from build123d import *

# Parameters (mm, degrees)
SKETCH1_W           = 28
SKETCH1_H           = 30
BOSS_EXTRUDE1_DEPTH = 12
SKETCH2_R           = 2.25
CUT_EXTRUDE1_DEPTH  = 36.213633723
SKETCH4_W           = 28
SKETCH4_H           = 15
CUT_EXTRUDE3_DEPTH  = 24.769728648
CUT_EXTRUDE4_DEPTH  = 5


with BuildPart() as part:
    # Sketch1 → Boss-Extrude1 (new body)
    with BuildSketch(Plane(origin=(0, 0, 0), x_dir=(1, 0, 0), z_dir=(0, 1, 0))):
        Rectangle(SKETCH1_W, SKETCH1_H)
        with BuildLine():
            Line((-1.590990258, -9.090990258), (0, -10.681980515))
            Line((0, -10.681980515), (1.590990258, -9.090990258))
            ThreePointArc((1.590990258, -9.090990258), (0, -5.25), (-1.590990258, -9.090990258))
        make_face(mode=Mode.SUBTRACT)
        with BuildLine():
            Line((-1.590990258, 5.909009742), (0, 4.318019485))
            Line((0, 4.318019485), (1.590990258, 5.909009742))
            ThreePointArc((1.590990258, 5.909009742), (0, 9.75), (-1.590990258, 5.909009742))
        make_face(mode=Mode.SUBTRACT)
    extrude(amount=BOSS_EXTRUDE1_DEPTH)

    # Sketch2 → Cut-Extrude1 (cut, through all)
    with BuildSketch(Plane.XY.offset(15)):
        with Locations((-9, 6)):
            Circle(SKETCH2_R)
        with Locations((9, 6)):
            Circle(SKETCH2_R)
    extrude(amount=-CUT_EXTRUDE1_DEPTH, mode=Mode.SUBTRACT)

    # Sketch4 → Cut-Extrude3 (cut, through all)
    with BuildSketch(Plane(origin=(0, 12, 0), x_dir=(1, 0, 0), z_dir=(0, 1, 0))):
        with Locations((0, -7.5)):
            Rectangle(SKETCH4_W, SKETCH4_H)
    extrude(amount=-CUT_EXTRUDE3_DEPTH, mode=Mode.SUBTRACT)

    # Sketch5 → Cut-Extrude4 (cut)
    with BuildSketch(Plane(origin=(0, 12, 0), x_dir=(1, 0, 0), z_dir=(0, 1, 0))):
        with BuildLine():
            Line((-2.828427125, 4.671572875), (0, 1.843145751))
            Line((0, 1.843145751), (2.828427125, 4.671572875))
            ThreePointArc((2.828427125, 4.671572875), (0, 11.5), (-2.828427125, 4.671572875))
        make_face()
    extrude(amount=-CUT_EXTRUDE4_DEPTH, mode=Mode.SUBTRACT)


solid = part.part
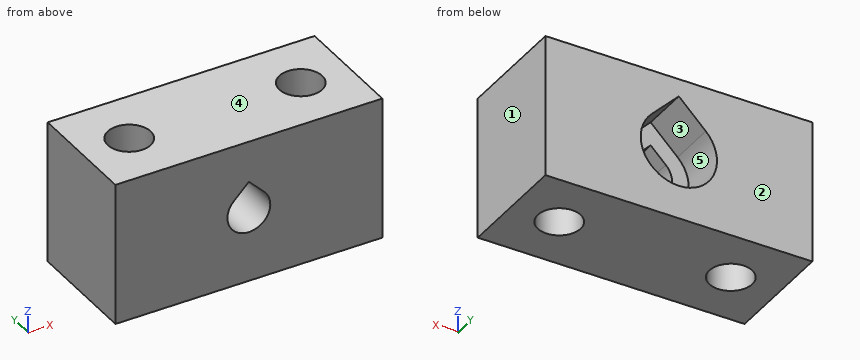
Here's how the part is built. I have some questions about the finished solid (model axes, mm). Face numbers are marked on the shaded views. A direction names the side the tool comes from. Give positions to 0.01 mm unless a question says otherwise; leave off trailing zeros. Order: outer loops, then holes, each group sorted by start corner. A loop starts at its lowest first (then second) coordinate and runs counter-clockwise, first axis right, second up. Notation, with made-up numbers: (-10, -27) -> (15, -27) arc R32 ccw to (15, 5) -> close; hole circle Ø9 at (23.25, 69.5). An arc over 180 degrees is marked (long way). Use a Markdown table: item, result. Add a question column.
Item 1: If we mould it in two halves opening along X, with no side actions, what happens to the marked faces 1, 2 and 3? For each: pulls with the +X half, pulls with the -X half, needs draft (parallel to the pull), parting line crosses it, or undercut.
Item 2: Imagine slicing it at D-D on z = -12.25. Please give me the cut outline in (x, y).
Item 3: Imagine slicing it at C-C on z = -7.5. Please give me the cut outline in (x, y).
Item 4: Will this pin go through, and if not, where does the flat tip stop? pin 1 (4 mm diameter, centred on x = 1, z = -6.5, fed in from +Y).
Item 5: Imagine slicing it at A-A on x = 9. Please give me the cut outline in (y, z), plus the area to 4 significant figures.
Item 6: I need wall thicknesses on line 1 (X direction, y = 10.55, z = -7.5); line 2 (X direction, y = 8, z = -14); line 3 (X direction, y = 5.25, z = -5.5). Which ranges of each line are inside material? Lowest first, please.
Item 7: For the marked faces 4 and 5, which set-ups out of +Z, -Z, +X, -X, +Y, -Y let a thin tool reach every point of the face, with its end or its side?
Item 8: Imagine slicing it at B-B on y = 4.25. Please give me the cut outline in (x, z).
Data:
| question | item | result |
|---|---|---|
| 1 | face 1 | pulls with the +X half |
| 1 | face 2 | needs draft |
| 1 | face 3 | undercut |
| 2 | outline | (-14, 0) -> (14, 0) -> (14, 12) -> (-14, 12) -> close; hole circle Ø4.5 at (-9, 6); hole circle Ø4.5 at (9, 6) |
| 3 | outline | (-14, 0) -> (-2.25, 0) -> (-2.25, 7) -> (-4, 7) -> (-4, 12) -> (-14, 12) -> close; (2.25, 0) -> (14, 0) -> (14, 12) -> (4, 12) -> (4, 7) -> (2.25, 7) -> close; hole circle Ø4.5 at (-9, 6); hole circle Ø4.5 at (9, 6) |
| 4 | pin 1 | stops at y = 7 |
| 5 | outline | (0, -15) -> (3.75, -15) -> (3.75, 0) -> (0, 0) -> close; (8.25, -15) -> (12, -15) -> (12, 0) -> (8.25, 0) -> close |
| 5 | area | 112.5 mm² |
| 6 | line 1 | x = -14 to -4, 4 to 14 |
| 6 | line 2 | x = -14 to -10.03, -7.97 to 7.97, 10.03 to 14 |
| 6 | line 3 | x = -14 to -11.12, -6.88 to -1.18, 1.18 to 6.88, 11.12 to 14 |
| 7 | face 4 | +Z, +X, -X, +Y, -Y |
| 7 | face 5 | +Y |
| 8 | outline | (-14, -15) -> (-10.41, -15) -> (-10.41, 0) -> (-14, 0) -> close; (-7.59, -15) -> (7.59, -15) -> (7.59, 0) -> (-7.59, 0) -> close; (10.41, -15) -> (14, -15) -> (14, 0) -> (10.41, 0) -> close; hole (-1.59, -5.91) arc R2.25 ccw (long way) to (1.59, -5.91) -> (0, -4.32) -> close |
